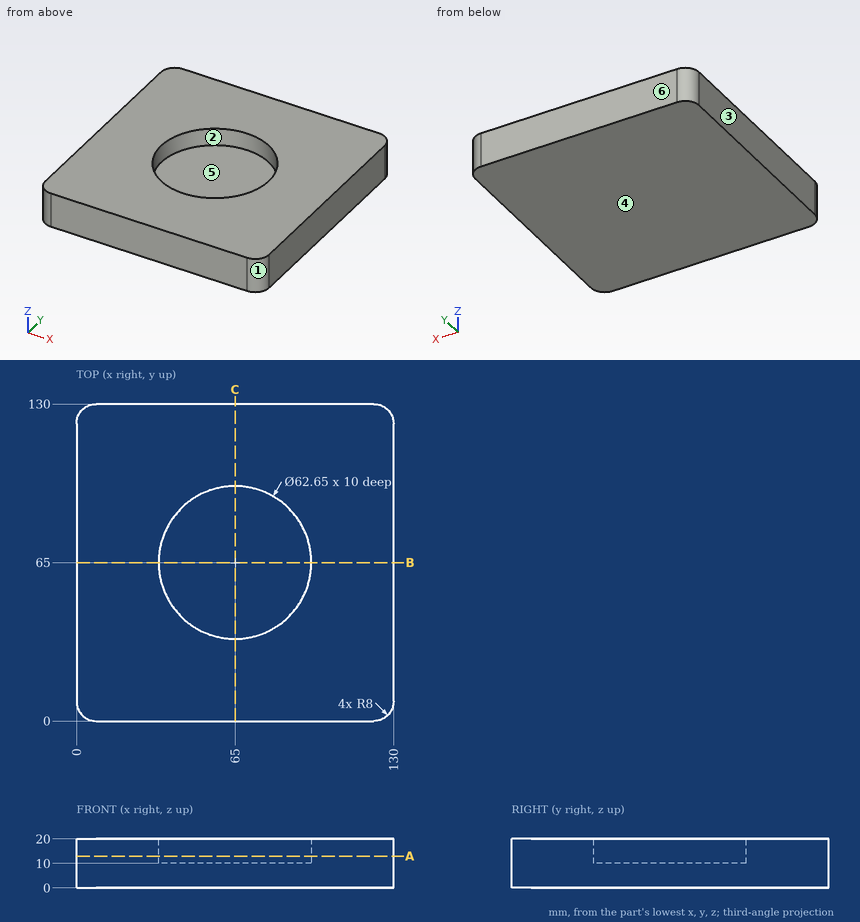
Source: three-view drawing plus pictorial views. Frame: mm from the lowest corner of the part. A direction names the side the tool comes from. Give positions to 0.01 mm unless a question says otherwise; leave off trailing zeros. Order: outer loops, then holes, each group sorted by start corner. A loop starts at its lowest first (then second) coordinate and runs counter-clockwise, first axis right, second up. Notation, with made-up numbers: M -9,63.25 L 27,63.25 A26 ccw 27,77.25 Z; hole C -1.5,-36.5 d3. An arc over 180 degrees is marked long. One line per question, with ' | ' between items.
1) Section B-B on y = 65. Output: boundary loops of the cut face in (x, z) (3 decimals).
Filled in:
outline: M 0,0 L 130,0 L 130,20 L 96.325,20 L 96.325,10 L 33.675,10 L 33.675,20 L 0,20 Z
2) Contact query for a flat-ended pin moving along its axis: P1, Ø2, axis at x = 92.5, y = 27, coming from the -Z side. Output: stop coordinate, or through.
Filled in:
P1: stops at z = 0
3) Access query for the marked faces 5 and 6. Directions: +Z, -Z, +X, -X, +Y, -Y. A direction counts if a zero-diameter tool reaches every point of the face in a straight line with its end or side. Return the directions, or none.
Filled in:
face 5: +Z | face 6: +Z, -Z, +X, -X, +Y
4) Section A-A on z = 13. Output: boundary loops of the cut face in (x, y) (3 decimals), and give its area (3 significant figures).
Filled in:
outline: M 0,8 A8 ccw 8,0 L 122,0 A8 ccw 130,8 L 130,122 A8 ccw 122,130 L 8,130 A8 ccw 0,122 Z; hole C 65,65 d62.65 | area: 13,800 mm2
5) Ray query, L1, parallel to Y at x = 65, z = 14.75 (3 decimals); L2, parallel to Y at x = 92, z = 10.25; L3, parallel to X at y = 88.5, z = 17. Return the intervals inside material, ascending.
Filled in:
L1: y = 0 to 33.675, 96.325 to 130 | L2: y = 0 to 49.12, 80.88 to 130 | L3: x = 0 to 44.29, 85.71 to 130
6) Draft query along X for the marked faces 1, 2, 3 and 4. Return one class per face: pulls with the +X half, pulls with the -X half, needs draft (parallel to the pull), parting line crosses it, or undercut.
Filled in:
face 1: pulls with the +X half | face 2: undercut | face 3: pulls with the -X half | face 4: needs draft
